Read the model definition and answer for the solid it produces. Units are mm, in the model's axes. Face numbers are marked on the shaded views. Round coordinates to 2 decimals unless told otherwise and drop trailing zeros. Write each loop counter-clockwise with the first axis right and the second up, starting at its lowest first coordinate (ties: lowest second). Pieces come first, ordered by that corner, then holes.
from build123d import *

# Parameters (mm, degrees)
ESQUISSE1_W             = 520
ESQUISSE1_H             = 520
BOSS_EXTRU_1_DEPTH      = 10
ESQUISSE2_W             = 480
ESQUISSE2_H             = 480
BOSS_EXTRU_2_DEPTH      = 10
ESQUISSE3_W             = 520
ESQUISSE3_H             = 520
ESQUISSE3_W_2           = 500
ESQUISSE3_H_2           = 500
BOSS_EXTRU_3_DEPTH      = 20
ESQUISSE4_R             = 25
ENL_V_MAT_EXTRU_1_DEPTH = 737.002717386


with BuildPart() as part:
    # Esquisse1 → Boss.-Extru.1 (new body)
    with BuildSketch(Plane.XY):
        with Locations((260, 260)):
            Rectangle(ESQUISSE1_W, ESQUISSE1_H)
    extrude(amount=BOSS_EXTRU_1_DEPTH)

    # Esquisse2 → Boss.-Extru.2 (add)
    with BuildSketch(Plane.XY.offset(10)):
        with Locations((260, 260)):
            Rectangle(ESQUISSE2_W, ESQUISSE2_H)
    extrude(amount=BOSS_EXTRU_2_DEPTH)

    # Esquisse3 → Boss.-Extru.3 (add)
    with BuildSketch(Plane.XY.offset(10)):
        with Locations((260, 260)):
            Rectangle(ESQUISSE3_W, ESQUISSE3_H)
        with Locations((260, 260)):
            Rectangle(ESQUISSE3_W_2, ESQUISSE3_H_2, mode=Mode.SUBTRACT)
    extrude(amount=BOSS_EXTRU_3_DEPTH)

    # Esquisse4 → Enlèv. mat.-Extru.1 (cut, through all)
    with BuildSketch(Plane(origin=(0, 0, 0), x_dir=(-1, 0, 0), z_dir=(0, 0, -1))):
        with Locations((-390, 110)):
            Circle(ESQUISSE4_R)
    extrude(amount=-ENL_V_MAT_EXTRU_1_DEPTH, mode=Mode.SUBTRACT)


solid = part.part
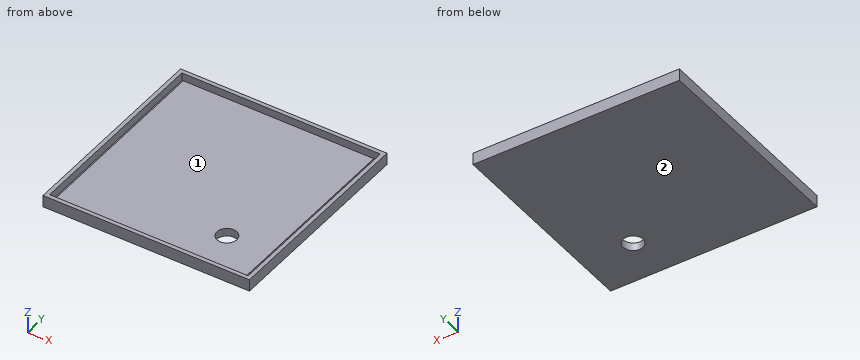
Q1. Section B-B (y = 110) is taken. Determine the outline of the cut face in (x, z), then the cut area to 3 significant figures.
Verdict:
outline: (0, 0) - (365, 0) - (365, 20) - (20, 20) - (20, 10) - (10, 10) - (10, 30) - (0, 30) - close; (415, 0) - (520, 0) - (520, 30) - (510, 30) - (510, 10) - (500, 10) - (500, 20) - (415, 20) - close
area: 9,400 mm2
Q2. Section C-C (x = 272.5) is taken. Determine the outline of the cut face in (y, z), then the cut area to 3 significant figures.
Verdict:
outline: (0, 0) - (520, 0) - (520, 30) - (510, 30) - (510, 10) - (500, 10) - (500, 20) - (20, 20) - (20, 10) - (10, 10) - (10, 30) - (0, 30) - close
area: 10,400 mm2
Q3. Determine the mould class of the marked faces 1 and 2 for opening direction Y: pulls with the +Y half, pulls with the -Y half, needs draft (parallel to the pull), parting line crosses it, or undercut.
Verdict:
face 1: undercut
face 2: needs draft
Q4. Flat-ended cylindrical pins translate along their axes: pin 1 Ø4 at (y, z) = (395.5, 16.5) entering from -X; pin 2 Ø8 at (x, y) = (260, 155) entering from +Z. Find the tip coordinate at first contact, or state that the pin passes through.
Verdict:
pin 1: stops at x = 0
pin 2: stops at z = 20
Q5. Straight lines are drawn through the part: probe 1 along X at (y, z) = (329, 15.5); probe 2 along Y at (x, z) = (390, 10.25); probe 3 along X at (y, z) = (490, 21). For each, find the intervals that lie inside material, in ascending order.
Verdict:
probe 1: x = 0 to 10, 20 to 500, 510 to 520
probe 2: y = 0 to 10, 20 to 85, 135 to 500, 510 to 520
probe 3: x = 0 to 10, 510 to 520
Q6. Section A-A (x = 390) is taken. Determine the outline of the cut face in (y, z), then the cut area to 3 significant figures.
Verdict:
outline: (0, 0) - (85, 0) - (85, 20) - (20, 20) - (20, 10) - (10, 10) - (10, 30) - (0, 30) - close; (135, 0) - (520, 0) - (520, 30) - (510, 30) - (510, 10) - (500, 10) - (500, 20) - (135, 20) - close
area: 9,400 mm2
